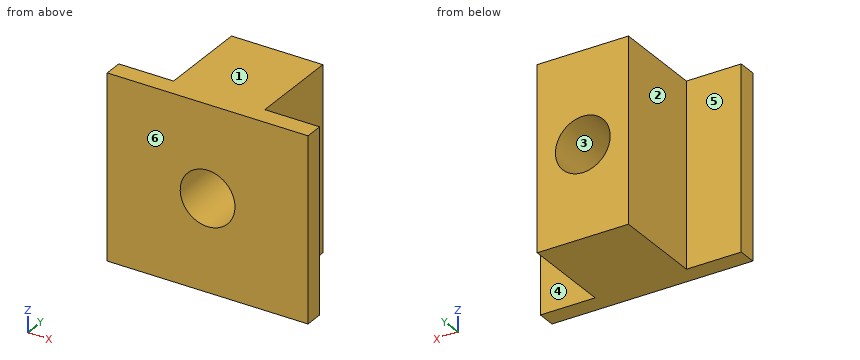
from build123d import *

# Parameters (mm, degrees)
SKETCH1_W           = 5
SKETCH1_H           = 10
BOSS_EXTRUDE1_DEPTH = 5
SKETCH2_W           = 11
SKETCH2_H           = 10
BOSS_EXTRUDE2_DEPTH = 1
SKETCH3_R           = 1.5
CUT_EXTRUDE1_DEPTH  = 10.552486587


with BuildPart() as part:
    # Sketch1 → Boss-Extrude1 (new body)
    with BuildSketch(Plane(origin=(0, 0, 0), x_dir=(1, 0, 0), z_dir=(0, 1, 0))):
        Rectangle(SKETCH1_W, SKETCH1_H)
    extrude(amount=BOSS_EXTRUDE1_DEPTH)

    # Sketch2 → Boss-Extrude2 (add)
    with BuildSketch(Plane.XZ):
        Rectangle(SKETCH2_W, SKETCH2_H)
    extrude(amount=BOSS_EXTRUDE2_DEPTH)

    # Sketch3 → Cut-Extrude1 (cut, through all)
    with BuildSketch(Plane.XZ.offset(1)):
        with Locations(Location((0, 0, 0), (0, 0, 270))):
            Circle(SKETCH3_R)
    extrude(amount=-CUT_EXTRUDE1_DEPTH, mode=Mode.SUBTRACT)


solid = part.part
The model under review builds one solid part; all positions refer to its coordinate system, in mm. Face numbers are marked on the shaded views. A direction names the side the tool comes from. Give positions to 0.01 mm unless a question says otherwise; leave off trailing zeros. Loops run counter-clockwise (first coordinate to the right, second up) from the corner with the lowest first, then second, coordinate; pieces in that order, holes last. Notation, with made-up numbers: (-26, 36) -> (33, 36) arc R25 cw to (33, 68) -> close; hole circle Ø3 at (15, -14). An arc over 180 degrees is marked (long way). Answer as a JSON object with one key per item and string values. Group by question number.
Q1. Take a section at D-D (z = -4). Write out the cut boundary in (x, y).
Q2. Wall thickness on line 1 along X through (y, z) = (0.7, 0); line 2 along Y through (x, z) = (3.75, 1.25); line 3 along Z through (x, y) = (0.25, 1.65): over which ranges is each line inside the solid? List them lowest first.
Q3. Take a section at B-B (z = 0). Write out the cut boundary in (x, y), plus the area to 3 significant figures.
Q4. Take a section at C-C (y = 3.95). Write out the cut boundary in (x, z), plus the area to 3 significant figures.
Q5. Take a section at A-A (x = 0). Write out the cut boundary in (y, z), plus the area to 3 significant figures.
Q6. Draft analysis for pull direction Z (two halves, no side actions). For the marked faces 1, 2 and 3, state which applies: pulls with the +Z half, pulls with the -Z half, needs draft (parallel to the pull), parting line crosses it, or undercut.
Q7. Tool access review of the marked faces 4, 5 and 6: name each direction out of +Z, -Z, +X, -X, +Y, -Y from which nothing blocks a thin tool from reaching the whole face with its end or side.
Q8. Insertion check: pin 1 (1.5 mm diameter, centred on x = -4, z = 0.5, fed in from +Y); pin 2 (2.5 mm diameter, centred on y = 3.5, z = 2, fed in from +X); pin 3 (2.5 mm diameter, centred on x = 0, z = 0, fed in from +Y). Each pin has a flat end and moves straight along its axis. Give the tip position at first contact, or say it passes through.
Answer below:
{
 "1": {"outline": "(-5.5, -1) -> (5.5, -1) -> (5.5, 0) -> (2.5, 0) -> (2.5, 5) -> (-2.5, 5) -> (-2.5, 0) -> (-5.5, 0) -> close"},
 "2": {"line 1": "x = -2.5 to -1.5, 1.5 to 2.5", "line 2": "y = -1 to 0", "line 3": "z = -5 to -1.48, 1.48 to 5"},
 "3": {"outline": "(-5.5, -1) -> (-1.5, -1) -> (-1.5, 5) -> (-2.5, 5) -> (-2.5, 0) -> (-5.5, 0) -> close; (1.5, -1) -> (5.5, -1) -> (5.5, 0) -> (2.5, 0) -> (2.5, 5) -> (1.5, 5) -> close", "area": "18.0 mm2"},
 "4": {"outline": "(-2.5, -5) -> (2.5, -5) -> (2.5, 5) -> (-2.5, 5) -> close; hole circle Ø3 at (0, 0)", "area": "42.9 mm2"},
 "5": {"outline": "(-1, -5) -> (5, -5) -> (5, -1.5) -> (-1, -1.5) -> close; (-1, 1.5) -> (5, 1.5) -> (5, 5) -> (-1, 5) -> close", "area": "42.0 mm2"},
 "6": {"face 1": "pulls with the +Z half", "face 2": "needs draft", "face 3": "undercut"},
 "7": {"face 4": "+Z, -Z, +X, +Y", "face 5": "+Z, -Z, -X, +Y", "face 6": "+Z, -Z, +X, -X, -Y"},
 "8": {"pin 1": "stops at y = 0", "pin 2": "stops at x = 2.5", "pin 3": "passes through"}
}
